Here's how the part is built. I have some questions about the finished solid (model axes, mm). A direction names the side the tool comes from. Round coordinates to 2 decimals unless told otherwise and drop trailing zeros. Loops run counter-clockwise (first coordinate to the right, second up) from the corner with the lowest first, then second, coordinate; pieces in that order, holes last. Notation, with made-up numbers: M 40.25,-7 L 98.25,-7 A10 ccw 98.25,-2 Z; hole C 16.25,2 d5. An arc over 180 degrees is marked long. Answer as a JSON object with one key per item and string values.
from build123d import *

# Parameters (mm, degrees)
SKETCH1_W            = 28
SKETCH1_H            = 22.8
BOSS_EXTRUDE1_DEPTH  = 48
SKETCH4_R            = 10.85
BOSS_EXTRUDE4_DEPTH  = 3.8
SKETCH5_R            = 9.9
BOSS_EXTRUDE5_DEPTH  = 12.1
SKETCH6_R            = 10.85
BOSS_EXTRUDE6_DEPTH  = 3.2
CUT_EXTRUDE3_DEPTH   = 1.8
FILLET2_R            = 1
FILLET2_OF_MIRROR2_R = 1
SKETCH9_W            = 25.4
SKETCH9_H            = 2.5
CUT_EXTRUDE4_DEPTH   = 25.8
FILLET3_R            = 1.5
SKETCH10_R           = 2.5
BOSS_EXTRUDE7_DEPTH  = 5.5
MIRROR6_START        = -12.2
MIRROR6_OUTLINE_W    = 1.3
MIRROR6_OUTLINE_H    = 22.8
MIRROR6_OUTLINE_W_2  = 44.2
MIRROR6_DEPTH        = 24.4
MIRROR6_START_2      = -14
MIRROR6_2_DEPTH      = 28
MIRROR6_START_3      = -19.5
MIRROR6_3_OUTLINE_R  = 2.5
MIRROR6_3_DEPTH      = 39
MIRROR6_START_4      = -12.5
MIRROR6_4_OUTLINE_W  = 1.3
MIRROR6_4_OUTLINE_H  = 22.8
MIRROR6_4_DEPTH      = 25
MIRROR6_START_5      = -11.4
MIRROR6_5_DEPTH      = 22.8


with BuildPart() as part:
    # Sketch1 → Boss-Extrude1 (new body)
    with BuildSketch(Plane(origin=(0, 0, 0), x_dir=(1, 0, 0), z_dir=(0, 1, 0))):
        Rectangle(SKETCH1_W, SKETCH1_H)
    extrude(amount=BOSS_EXTRUDE1_DEPTH)

    # Sketch4 → Boss-Extrude4 (add)
    with BuildSketch(Plane.XZ):
        with Locations(Location((0, 0, 0), (0, 0, 90))):
            Circle(SKETCH4_R)
    extrude(amount=BOSS_EXTRUDE4_DEPTH)

    # Sketch5 → Boss-Extrude5 (add)
    with BuildSketch(Plane.XZ.offset(3.8)):
        with Locations(Location((0, 0, 0), (0, 0, 270))):
            Circle(SKETCH5_R)
    extrude(amount=BOSS_EXTRUDE5_DEPTH)

    # Sketch6 → Boss-Extrude6 (add)
    with BuildSketch(Plane.XZ.offset(15.9)):
        with Locations(Location((0, 0, 0), (0, 0, 90))):
            Circle(SKETCH6_R)
    extrude(amount=BOSS_EXTRUDE6_DEPTH)

    # Sketch8 → Cut-Extrude3 (cut)
    with BuildSketch(Plane(origin=(14, 0, 0), x_dir=(0, 0, -1), z_dir=(1, 0, 0))):
        with BuildLine():
            Line((8.6, 8.6), (11.4, 8.6))
            Line((11.4, 8.6), (11.4, 48))
            Line((11.4, 48), (-11.4, 48))
            Line((-11.4, 48), (-11.4, 8.6))
            Line((-11.4, 8.6), (-8.6, 8.6))
            Line((-8.6, 8.6), (-8.6, 25.4))
            ThreePointArc((-8.6, 25.4), (-6.4, 27.6), (-8.6, 29.8))
            Line((-8.6, 29.8), (-8.6, 43))
            ThreePointArc((-8.6, 43), (-7.044365081, 43.644365081), (-6.4, 45.2))
            Line((-6.4, 45.2), (6.4, 45.2))
            ThreePointArc((6.4, 45.2), (7.044365081, 43.644365081), (8.6, 43))
            Line((8.6, 43), (8.6, 29.8))
            ThreePointArc((8.6, 29.8), (6.4, 27.6), (8.6, 25.4))
            Line((8.6, 25.4), (8.6, 8.6))
        make_face()
    cut_extrude3 = extrude(amount=-CUT_EXTRUDE3_DEPTH, mode=Mode.SUBTRACT)

    # Fillet2
    fillet2_edges = [part.edges().sort_by_distance(p)[0] for p in [
        (13.1, 8.6, 11.4),
        (13.1, 8.6, -11.4),
    ]]
    fillet(fillet2_edges, radius=FILLET2_R)

    # Mirror2: Cut-Extrude3 across plane
    add(cut_extrude3.mirror(Plane(origin=(0, 0, 0), x_dir=(0, 0, 1), z_dir=(1, 0, 0))), mode=Mode.SUBTRACT)

    # Fillet2 of Mirror2
    fillet2_of_mirror2_edges = [part.edges().sort_by_distance(p)[0] for p in [
        (-13.1, 8.6, 11.4),
        (-13.1, 8.6, -11.4),
    ]]
    fillet(fillet2_of_mirror2_edges, radius=FILLET2_OF_MIRROR2_R)

    # Sketch9 → Cut-Extrude4 (cut)
    with BuildSketch(Plane(origin=(0, 0, -11.4), x_dir=(-1, 0, 0), z_dir=(0, 0, -1))):
        with Locations((0, 2.55)):
            Rectangle(SKETCH9_W, SKETCH9_H)
    extrude(amount=-CUT_EXTRUDE4_DEPTH, mode=Mode.SUBTRACT)

    # Fillet3
    fillet3_edges = [part.edges().sort_by_distance(p)[0] for p in [
        (12.7, 1.3, 0),
        (-12.7, 1.3, 0),
        (-14, 0, 0),
        (14, 0, 0),
    ]]
    fillet(fillet3_edges, radius=FILLET3_R)

    # Sketch10 → Boss-Extrude7 (add)
    with BuildSketch(Plane.ZY.offset(14)):
        with Locations(Location((0, 34.2, 0), (0, 0, 180))):
            Circle(SKETCH10_R)
    boss_extrude7 = extrude(amount=BOSS_EXTRUDE7_DEPTH)

    # Mirror3: Boss-Extrude7 across plane
    add(boss_extrude7.mirror(Plane(origin=(0, 0, 0), x_dir=(0, 0, 1), z_dir=(1, 0, 0))))

    # Mirror6: read off the stored shape, not the designer's step
    # Mirror6 outline → Mirror6 (add)
    with BuildSketch(Plane.YZ.offset(MIRROR6_START)):
        with Locations((-19.75, 0)):
            Rectangle(MIRROR6_OUTLINE_W, MIRROR6_OUTLINE_H)
        with Locations((-45, 0)):
            Rectangle(MIRROR6_OUTLINE_W_2, MIRROR6_OUTLINE_H)
    extrude(amount=MIRROR6_DEPTH)

    # Mirror6 2 outline → Mirror6 2 (add)
    with BuildSketch(Plane.YZ.offset(MIRROR6_START_2)):
        with BuildLine():
            Line((-26.7, -11.4), (-22.9, -11.4))
            Line((-22.9, -11.4), (-22.9, 11.4))
            Line((-22.9, 11.4), (-26.7, 11.4))
            ThreePointArc((-26.7, 11.4), (-27.407106781, 11.107106781), (-27.7, 10.4))
            Line((-27.7, 10.4), (-27.7, 8.6))
            Line((-27.7, 8.6), (-44.5, 8.6))
            ThreePointArc((-44.5, 8.6), (-46.7, 6.4), (-48.9, 8.6))
            Line((-48.9, 8.6), (-62.1, 8.6))
            ThreePointArc((-62.1, 8.6), (-62.744365081, 7.044365081), (-64.3, 6.4))
            Line((-64.3, 6.4), (-64.3, -6.4))
            ThreePointArc((-64.3, -6.4), (-62.744365081, -7.044365081), (-62.1, -8.6))
            Line((-62.1, -8.6), (-48.9, -8.6))
            ThreePointArc((-48.9, -8.6), (-46.7, -6.4), (-44.5, -8.6))
            Line((-44.5, -8.6), (-27.7, -8.6))
            Line((-27.7, -8.6), (-27.7, -10.4))
            ThreePointArc((-27.7, -10.4), (-27.407106781, -11.107106781), (-26.7, -11.4))
        make_face()
    extrude(amount=MIRROR6_2_DEPTH)

    # Mirror6 3 outline → Mirror6 3 (add)
    with BuildSketch(Plane.YZ.offset(MIRROR6_START_3)):
        with Locations((-53.3, 0)):
            Circle(MIRROR6_3_OUTLINE_R)
    extrude(amount=MIRROR6_3_DEPTH)

    # Mirror6 4 outline → Mirror6 4 (add)
    with BuildSketch(Plane.YZ.offset(MIRROR6_START_4)):
        with Locations((-19.75, 0)):
            Rectangle(MIRROR6_4_OUTLINE_W, MIRROR6_4_OUTLINE_H)
    extrude(amount=MIRROR6_4_DEPTH)

    # Mirror6 5 outline → Mirror6 5 (add)
    with BuildSketch(Plane.XY.offset(MIRROR6_START_5)):
        with BuildLine():
            Line((12.7, -21.9), (12.7, -22.9))
            Line((12.7, -22.9), (14, -22.9))
            Line((14, -22.9), (14, -20.6))
            ThreePointArc((14, -20.6), (13.560660172, -19.539339828), (12.5, -19.1))
            Line((12.5, -19.1), (12.5, -20.4))
            Line((12.5, -20.4), (11.2, -20.4))
            ThreePointArc((11.2, -20.4), (12.260660172, -20.839339828), (12.7, -21.9))
        make_face()
        with BuildLine():
            Line((-14, -22.9), (-12.7, -22.9))
            Line((-12.7, -22.9), (-12.7, -21.9))
            ThreePointArc((-12.7, -21.9), (-12.260660172, -20.839339828), (-11.2, -20.4))
            Line((-11.2, -20.4), (-12.5, -20.4))
            Line((-12.5, -20.4), (-12.5, -19.1))
            ThreePointArc((-12.5, -19.1), (-13.560660172, -19.539339828), (-14, -20.6))
            Line((-14, -20.6), (-14, -22.9))
        make_face()
    extrude(amount=MIRROR6_5_DEPTH)


solid = part.part
Item 1: If I drill on L1, parallel to Y at x = 8, z = 5.5; L2, parallel to Y at x = 10.5, z = -6; L3, parallel to Y at x = 6, z = -8.5, over which ranges is the centre line in solid material (lowest first)? Write a range as from..to.
Solution:
{"L1": "y = -67.1..-22.9, -20.4..1.3, 3.8..48", "L2": "y = -67.1..-22.9, -20.4..-19.1, 0..1.3, 3.8..48", "L3": "y = -67.1..-22.9, -20.4..-15.9, -3.8..1.3, 3.8..48"}
Item 2: I want a section at A-A on x = 8. List the corners of the cut face in (y, z) for me.
Solution:
{"outline": "M -67.1,-11.4 L -22.9,-11.4 L -22.9,11.4 L -67.1,11.4 Z; M -20.4,-11.4 L -19.1,-11.4 L -19.1,-7.33 L -15.9,-7.33 L -15.9,-5.83 L -3.8,-5.83 L -3.8,-7.33 L 0,-7.33 L 0,-11.4 L 1.3,-11.4 L 1.3,11.4 L 0,11.4 L 0,7.33 L -3.8,7.33 L -3.8,5.83 L -15.9,5.83 L -15.9,7.33 L -19.1,7.33 L -19.1,11.4 L -20.4,11.4 Z; M 3.8,-11.4 L 48,-11.4 L 48,11.4 L 3.8,11.4 Z"}
Item 3: For P1, Ø10, axis at x = 4, y = -10.5, coming from the -Z side; P2, Ø1.1, axis at y = 3.5, z = 2, coming from the +X side; P3, Ø0.5, axis at x = 13, y = 37.5, coming from the +Z side; P4, Ø5, axis at x = -14.5, y = 1, coming from the +Z side, each with a flat end and sliding along its axis, tell me the tip position at first contact or that it passes through.
Solution:
{"P1": "stops at z = -9.9", "P2": "stops at x = 14", "P3": "stops at z = 8.6", "P4": "stops at z = 11.4"}
Item 4: I want a section at B-B on y = -39.5. List the corners of the cut face in (x, z) for me, plus the area to 3 significant figures.
Solution:
{"outline": "M -14,-8.6 L -12.2,-8.6 L -12.2,-11.4 L 12.2,-11.4 L 12.2,-8.6 L 14,-8.6 L 14,8.6 L 12.2,8.6 L 12.2,11.4 L -12.2,11.4 L -12.2,8.6 L -14,8.6 Z", "area": "618 mm2"}
Item 5: I want a section at D-D on y = 34.2. List the corners of the cut face in (x, z) for me, plus the area to 3 significant figures.
Solution:
{"outline": "M -19.5,-2.5 L -14,-2.5 L -14,-8.6 L -12.2,-8.6 L -12.2,-11.4 L 12.2,-11.4 L 12.2,-8.6 L 14,-8.6 L 14,-2.5 L 19.5,-2.5 L 19.5,2.5 L 14,2.5 L 14,8.6 L 12.2,8.6 L 12.2,11.4 L -12.2,11.4 L -12.2,8.6 L -14,8.6 L -14,2.5 L -19.5,2.5 Z", "area": "673 mm2"}
Item 6: We'd pull the mould along X, two halves only. Please class faces 4 (the face through (19.5, -53, 0)), 5 (the face through (2.974, -9.765, -9.443)), 6 (the face through (0, -43, -11.4)), 7 (the face through (0, -22.9, 0)): +X half, -X half, draft (parallel to the pull), parting line (faces both ways), or undercut.
Solution:
{"face 4": "+X half", "face 5": "parting line", "face 6": "draft", "face 7": "undercut"}
Item 7: I want a section at C-C on x = -15. List the corners of the cut face in (y, z) for me, plus the area to 3 significant figures.
Solution:
{"outline": "C -53.3,0 d5; C 34.2,0 d5", "area": "39.3 mm2"}
Item 8: For faces 1 (the face through (13.09, -62.76, -7.03)), 2 (the face through (-13.1, 27.6, -6.4)), 3 (the face through (-13.11, -62.76, -7.03)), which set-ups out of +Z, -Z, +X, -X, +Y, -Y let a thin tool reach every point of the face, with its end or its side?
Solution:
{"face 1": "-Z, +X, -Y", "face 2": "-Z, -X", "face 3": "-Z, -X, -Y"}
